CAD build for the part. Positions are in the model's coordinates, mm. A direction names the side the tool comes from. Round coordinates to 2 decimals unless told otherwise and drop trailing zeros. Order: outer loops, then holes, each group sorted by start corner. A loop starts at its lowest first (then second) coordinate and runs counter-clockwise, first axis right, second up. Notation, with made-up numbers: M -2,2 L 20,2 A11 cw 20,15 Z; hole C -23,8.5 d5. An arc over 180 degrees is marked long. Answer as a JSON object with one key per item and string values.
```python
from build123d import *

# Parameters (mm, degrees)
SKETCH1_W            = 45
SKETCH1_H            = 100
BOSS_EXTRUDE1_DEPTH  = 2.70166895
SKETCH2_R            = 1.5
CUT_EXTRUDE1_DEPTH   = 2.70166895
LPATTERN1_COUNT      = 2
LPATTERN1_PITCH      = 85
LPATTERN1_COUNT_DIR2 = 2
LPATTERN1_PITCH_DIR2 = 34.4
SKETCH4_W            = 30
SKETCH4_H            = 2.70166895
BOSS_EXTRUDE2_DEPTH  = 10
SKETCH6_W            = 3
SKETCH6_H            = 30
BOSS_EXTRUDE3_DEPTH  = 20
SKETCH7_W            = 30
SKETCH7_H            = 2.5
BOSS_EXTRUDE4_DEPTH  = 7.5
SKETCH14_W           = 3
SKETCH14_H           = 30
BOSS_EXTRUDE5_DEPTH  = 20
SKETCH15_W           = 30
SKETCH15_H           = 2.5
BOSS_EXTRUDE6_DEPTH  = 7.5
SKETCH16_R           = 1.5
CUT_EXTRUDE2_DEPTH   = 2.5
LPATTERN2_COUNT      = 2
LPATTERN2_PITCH      = 22
LPATTERN2_COUNT_DIR2 = 2
LPATTERN2_PITCH_DIR2 = 72


with BuildPart() as part:
    # Sketch1 → Boss-Extrude1 (new body)
    with BuildSketch(Plane(origin=(0, 0, 0), x_dir=(1, 0, 0), z_dir=(0, 1, 0))):
        with Locations((-22.5, 50)):
            Rectangle(SKETCH1_W, SKETCH1_H)
    extrude(amount=BOSS_EXTRUDE1_DEPTH)

    # Sketch2 → Cut-Extrude1 (cut)
    with BuildSketch(Plane(origin=(0, 2.70166895, 0), x_dir=(1, 0, 0), z_dir=(0, 1, 0))):
        with Locations(Location((-39.7, 92.5, 0), (0, 0, 270))):
            Circle(SKETCH2_R)
    cut_extrude1 = extrude(amount=-CUT_EXTRUDE1_DEPTH, mode=Mode.SUBTRACT)

    # LPattern1: Cut-Extrude1 2 × 2
    with Locations(*[(j * LPATTERN1_PITCH_DIR2, 0, i * LPATTERN1_PITCH) for i in range(LPATTERN1_COUNT) for j in range(LPATTERN1_COUNT_DIR2) if (i, j) != (0, 0)]):
        add(cut_extrude1, mode=Mode.SUBTRACT)

    # Sketch4 → Boss-Extrude2 (add)
    with BuildSketch(Plane(origin=(0, 0, 0), x_dir=(0, 0, -1), z_dir=(1, 0, 0))):
        with Locations((50, 1.350834475)):
            Rectangle(SKETCH4_W, SKETCH4_H)
    boss_extrude2 = extrude(amount=BOSS_EXTRUDE2_DEPTH)

    # Sketch6 → Boss-Extrude3 (add)
    with BuildSketch(Plane.XZ):
        with Locations((8.5, -50)):
            Rectangle(SKETCH6_W, SKETCH6_H)
    extrude(amount=BOSS_EXTRUDE3_DEPTH)

    # Sketch7 → Boss-Extrude4 (add)
    with BuildSketch(Plane(origin=(10, 0, 0), x_dir=(0, 0, -1), z_dir=(1, 0, 0))):
        with Locations((50, -18.75)):
            Rectangle(SKETCH7_W, SKETCH7_H)
    extrude(amount=BOSS_EXTRUDE4_DEPTH)

    # Mirror2: Boss-Extrude2 across plane
    add(boss_extrude2.mirror(Plane.ZY.offset(22.5)))

    # Sketch14 → Boss-Extrude5 (add)
    with BuildSketch(Plane.XZ):
        with Locations((-53.5, -50)):
            Rectangle(SKETCH14_W, SKETCH14_H)
    extrude(amount=BOSS_EXTRUDE5_DEPTH)

    # Sketch15 → Boss-Extrude6 (add)
    with BuildSketch(Plane.ZY.offset(55)):
        with Locations((-50, -18.75)):
            Rectangle(SKETCH15_W, SKETCH15_H)
    extrude(amount=BOSS_EXTRUDE6_DEPTH)

    # Sketch16 → Cut-Extrude2 (cut)
    with BuildSketch(Plane(origin=(0, -17.5, 0), x_dir=(1, 0, 0), z_dir=(0, 1, 0))):
        with Locations(Location((-58.5, 61, 0), (0, 0, 270))):
            Circle(SKETCH16_R)
    cut_extrude2 = extrude(amount=-CUT_EXTRUDE2_DEPTH, mode=Mode.SUBTRACT)

    # LPattern2: Cut-Extrude2 2 × 2
    with Locations(*[(j * LPATTERN2_PITCH_DIR2, 0, i * LPATTERN2_PITCH) for i in range(LPATTERN2_COUNT) for j in range(LPATTERN2_COUNT_DIR2) if (i, j) != (0, 0)]):
        add(cut_extrude2, mode=Mode.SUBTRACT)


solid = part.part
```
Item 1: Saw through at C-C on x = 13.5. List the corners of the cut face in (y, z), and give its area (3 significant figures).
Worked answers:
{"outline": "M -20,-65 L -17.5,-65 L -17.5,-62.5 L -20,-62.5 Z; M -20,-59.5 L -17.5,-59.5 L -17.5,-40.5 L -20,-40.5 Z; M -20,-37.5 L -17.5,-37.5 L -17.5,-35 L -20,-35 Z", "area": "60.0 mm2"}
Item 2: Saw through at B-B on y = -12.75. List the corners of the cut face in (x, z).
Worked answers:
{"outline": "M -55,-65 L -52,-65 L -52,-35 L -55,-35 Z; M 7,-65 L 10,-65 L 10,-35 L 7,-35 Z"}
Item 3: 3-axis set-ups, long thin cutter, end or side, ignore diameter. For faces 1 (the flat face through (8, -9, -35)), 2 (the flat face through (-45, 1, -17)), 3 (the flat face through (8, -9, -65)): which of +Z, -Z, +X, -X, +Y, -Y reach the whole face in a straight line?
Worked answers:
{"face 1": "+Z, +X, +Y, -Y", "face 2": "+Z, -X, +Y, -Y", "face 3": "-Z, +X, +Y, -Y"}
Item 4: Wall check: line 1 along X through (y, z) = (1.5, -92.5); line 2 along X through (y, z) = (-18.35, -61); line 3 along X through (y, z) = (-18.25, -46). Give the ranges that are in metal, low to high. Write a range as [from, to].
Worked answers:
{"line 1": "x = [-45, -41.2], [-38.2, -6.8], [-3.8, 0]", "line 2": "x = [-62.5, -60], [-57, -52], [7, 12], [15, 17.5]", "line 3": "x = [-62.5, -52], [7, 17.5]"}
Item 5: Drop flat-ended pins along their axis: pin 1 Ø10 at (y, z) = (-8, -54.5) entering from -X; pin 2 Ø6 at (x, z) = (-22, -14) entering from -Y; pin 3 Ø4 at (x, z) = (15.5, -49) entering from +Y. Give the stop position or say it passes through.
Worked answers:
{"pin 1": "stops at x = -55", "pin 2": "stops at y = 0", "pin 3": "stops at y = -17.5"}
Item 6: Two-plate mould, pull along X, no slides. Class faces 4 (the flat face through (-59, -17.5, -50)), 5 (the cylindrical face through (-57.49, -18.73, -40.11)), 6 (the flat face through (0, 1, -17)): released by +X, released by -X, zero draft, split by the parting line, or undercut.
Worked answers:
{"face 4": "zero draft", "face 5": "undercut", "face 6": "released by +X"}
Item 7: Saw through at D-D on z = -7.5. List the corners of the cut face in (x, y), and give its area (3 significant figures).
Worked answers:
{"outline": "M -45,0 L -41.2,0 L -41.2,2.7 L -45,2.7 Z; M -38.2,0 L -6.8,0 L -6.8,2.7 L -38.2,2.7 Z; M -3.8,0 L 0,0 L 0,2.7 L -3.8,2.7 Z", "area": "105 mm2"}
Item 8: Saw through at A-A on z = -61. List the corners of the cut face in (x, y).
Worked answers:
{"outline": "M -62.5,-20 L -60,-20 L -60,-17.5 L -62.5,-17.5 Z; M -57,-20 L -52,-20 L -52,0 L 7,0 L 7,-20 L 12,-20 L 12,-17.5 L 10,-17.5 L 10,2.7 L -55,2.7 L -55,-17.5 L -57,-17.5 Z; M 15,-20 L 17.5,-20 L 17.5,-17.5 L 15,-17.5 Z"}
